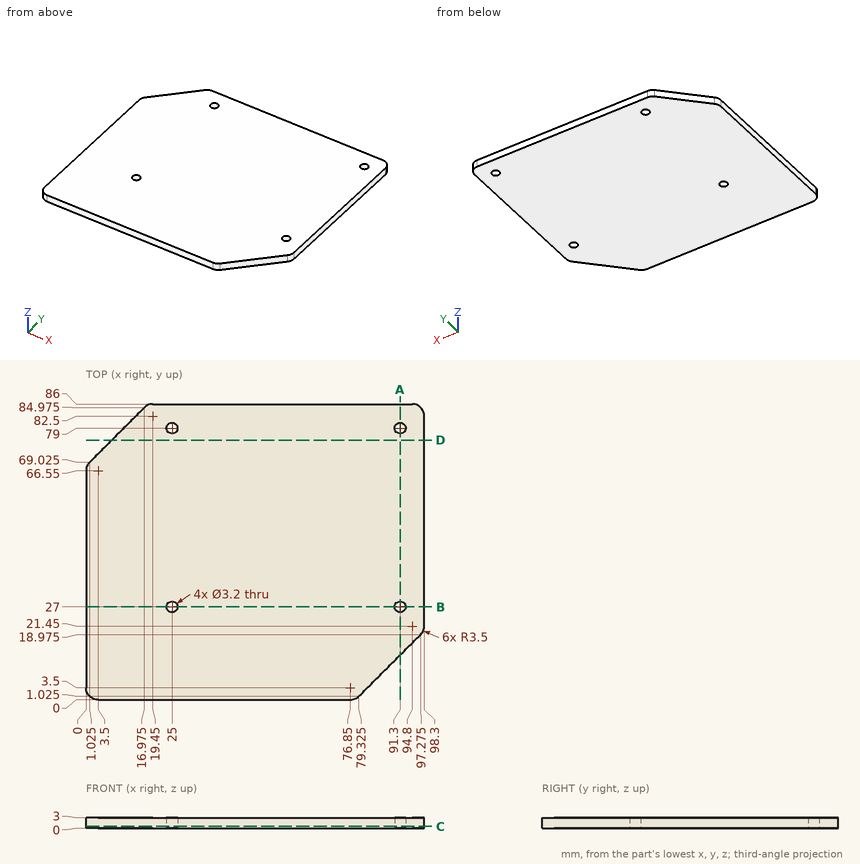
Can you work these out from the drawing? Everything is in mm from the part's minimum corner. Coordinates: 2 decimals unless noted, no trailing zeros. Write each loop counter-clockwise with the first axis right and the second up, starting at its lowest first coordinate (ties: lowest second). Pieces come first, ordered by that corner, then holes. Notation, with made-up numbers: (-16.75, -9) -> (26.25, -9) arc R29 cw to (26.25, 29) -> close; hole circle Ø5 at (-4, -18.5). An arc over 180 degrees is marked (long way). Write each question's results on one line, items separated by ' | '. Start each with the question number.
Item 1: I'm going to push a flat-ended pin straight in: P1, Ø1.5, axis at x = 87.5, z = 1.5, coming from the -Y side. Where does the tip first touch, or does it pass through?
Item 2: If we section it at A-A, the plane x = 91.3: Write out the boundary of the cut face in (y, z), and give its area (3 significant figures).
Item 3: Please list where these lines run through material, in increasing order: probe 1 along Y at (x, z) = (25, 0.7); probe 2 along Y at (x, z) = (91.3, 1.1); probe 3 along X at (y, z) = (79, 1.95).
Item 4: If we section it at B-B, the plane y = 27: Write out the boundary of the cut face in (x, z), and give its area (3 significant figures).
Item 5: If we section it at C-C, the plane z = 0.55: Count the separate pieces of the cut face and the enclosed holes in it, and give its area (3 significant figures).
Item 6: If we section it at D-D, the plane y = 75.5: Write out the boundary of the cut face in (x, z), and give its area (3 significant figures).
Answer block:
1) P1: y = 8.45
2) outline: (13, 0) -> (25.4, 0) -> (25.4, 3) -> (13, 3) -> close; (28.6, 0) -> (77.4, 0) -> (77.4, 3) -> (28.6, 3) -> close; (80.6, 0) -> (86, 0) -> (86, 3) -> (80.6, 3) -> close | area: 200 mm²
3) probe 1: 0 to 25.4, 28.6 to 77.4, 80.6 to 86 | probe 2: 13 to 25.4, 28.6 to 77.4, 80.6 to 86 | probe 3: 11 to 23.4, 26.6 to 89.7, 92.9 to 98.3
4) outline: (0, 0) -> (23.4, 0) -> (23.4, 3) -> (0, 3) -> close; (26.6, 0) -> (89.7, 0) -> (89.7, 3) -> (26.6, 3) -> close; (92.9, 0) -> (98.3, 0) -> (98.3, 3) -> (92.9, 3) -> close | area: 276 mm²
5) separate pieces: 1 | enclosed holes: 4 | area: 8,050 mm²
6) outline: (7.5, 0) -> (98.3, 0) -> (98.3, 3) -> (7.5, 3) -> close | area: 272 mm²
